Read the model definition and answer for the solid it produces. Units are mm, in the model's axes. Coordinates: 2 decimals unless noted, no trailing zeros. Write each loop counter-clockwise with the first axis right and the second up, starting at its lowest first coordinate (ties: lowest second). Pieces come first, ordered by that corner, then holes. Notation, with made-up numbers: (-2, -29) -> (14, -29) arc R18 cw to (14, -16) -> close; hole circle Ø2 at (87.5, 14.5). An arc over 180 degrees is marked (long way). Return JSON: item names as keys, results as strings.
from build123d import *

# Parameters (mm, degrees)
F0_R     = 22.5
F0_R_2   = 4
F1_DEPTH = 6


with BuildPart() as f1:
    # F0 (on Front) → F1 (new body)
    with BuildSketch(Plane.XZ):
        Circle(F0_R)
        with BuildLine():
            ThreePointArc((12.788895, 9.614789), (14.782073, 6.122935), (15.841797, 2.244431))
            ThreePointArc((15.841797, 2.244431), (17.534038, 1.645973), (18.25, 0))
            ThreePointArc((18.25, 0), (17.534038, -1.645973), (15.841797, -2.244431))
            ThreePointArc((15.841797, -2.244431), (14.782073, -6.122935), (12.788895, -9.614789))
            ThreePointArc((12.788895, -9.614789), (13.360861, -10.380078), (13.563708, -11.313708))
            ThreePointArc((13.563708, -11.313708), (12.101088, -13.42144), (9.614789, -12.788895))
            ThreePointArc((9.614789, -12.788895), (6.122935, -14.782073), (2.244431, -15.841797))
            ThreePointArc((2.244431, -15.841797), (2.248607, -15.920849), (2.25, -16))
            ThreePointArc((2.25, -16), (-0.079151, -18.248607), (-2.244431, -15.841797))
            ThreePointArc((-2.244431, -15.841797), (-6.122935, -14.782073), (-9.614789, -12.788895))
            ThreePointArc((-9.614789, -12.788895), (-12.904699, -12.904699), (-12.788895, -9.614789))
            ThreePointArc((-12.788895, -9.614789), (-14.782073, -6.122935), (-15.841797, -2.244431))
            ThreePointArc((-15.841797, -2.244431), (-18.25, 0), (-15.841797, 2.244431))
            ThreePointArc((-15.841797, 2.244431), (-14.782073, 6.122935), (-12.788895, 9.614789))
            ThreePointArc((-12.788895, 9.614789), (-12.904699, 12.904699), (-9.614789, 12.788895))
            ThreePointArc((-9.614789, 12.788895), (-6.122935, 14.782073), (-2.244431, 15.841797))
            ThreePointArc((-2.244431, 15.841797), (-0.079151, 18.248607), (2.25, 16))
            ThreePointArc((2.25, 16), (2.248607, 15.920849), (2.244431, 15.841797))
            ThreePointArc((2.244431, 15.841797), (6.122935, 14.782073), (9.614789, 12.788895))
            ThreePointArc((9.614789, 12.788895), (12.101088, 13.42144), (13.563708, 11.313708))
            ThreePointArc((13.563708, 11.313708), (13.360861, 10.380078), (12.788895, 9.614789))
        make_face(mode=Mode.SUBTRACT)
        with BuildLine():
            ThreePointArc((15.841797, -2.244431), (13.75, 0), (15.841797, 2.244431))
            ThreePointArc((15.841797, 2.244431), (14.782073, 6.122935), (12.788895, 9.614789))
            ThreePointArc((12.788895, 9.614789), (9.722718, 9.722718), (9.614789, 12.788895))
            ThreePointArc((9.614789, 12.788895), (6.122935, 14.782073), (2.244431, 15.841797))
            ThreePointArc((2.244431, 15.841797), (0, 13.75), (-2.244431, 15.841797))
            ThreePointArc((-2.244431, 15.841797), (-6.122935, 14.782073), (-9.614789, 12.788895))
            ThreePointArc((-9.614789, 12.788895), (-9.205977, 12.101088), (-9.063708, 11.313708))
            ThreePointArc((-9.063708, 11.313708), (-10.380078, 9.266556), (-12.788895, 9.614789))
            ThreePointArc((-12.788895, 9.614789), (-14.782073, 6.122935), (-15.841797, 2.244431))
            ThreePointArc((-15.841797, 2.244431), (-14.354027, 1.534038), (-13.75, 0))
            ThreePointArc((-13.75, 0), (-14.354027, -1.534038), (-15.841797, -2.244431))
            ThreePointArc((-15.841797, -2.244431), (-14.782073, -6.122935), (-12.788895, -9.614789))
            ThreePointArc((-12.788895, -9.614789), (-10.380078, -9.266556), (-9.063708, -11.313708))
            ThreePointArc((-9.063708, -11.313708), (-9.205977, -12.101088), (-9.614789, -12.788895))
            ThreePointArc((-9.614789, -12.788895), (-6.122935, -14.782073), (-2.244431, -15.841797))
            ThreePointArc((-2.244431, -15.841797), (0, -13.75), (2.244431, -15.841797))
            ThreePointArc((2.244431, -15.841797), (6.122935, -14.782073), (9.614789, -12.788895))
            ThreePointArc((9.614789, -12.788895), (9.722718, -9.722718), (12.788895, -9.614789))
            ThreePointArc((12.788895, -9.614789), (14.782073, -6.122935), (15.841797, -2.244431))
        make_face()
        Circle(F0_R_2, mode=Mode.SUBTRACT)
    extrude(amount=F1_DEPTH)


solid = f1.part
1. For a pull along Z with two mould halves and no side action, classify faces 1 (the face through (-9.2, -2.96, -12.09)), 2 (the face through (0, -6, -5)), 3 (the face through (10.382, -2.958, -19.961)), 4 (the face through (-9.21, -2.96, 12.11)) as +Z half, -Z half, draft (parallel to the pull), parting line (faces both ways), or undercut.
Taken from the geometry:
{"face 1": "undercut", "face 2": "draft", "face 3": "parting line", "face 4": "undercut"}
2. Consider L1, parallel to Z at x = 0, y = -1.85; L2, parallel to X at y = -0.9, z = 12; L3, parallel to X at y = -2.3, z = -1. Determine where each line is inside the solid, lowest interval first.
Taken from the geometry:
{"L1": "z = -22.5 to -18.25, -13.75 to -4, 4 to 13.75, 18.25 to 22.5", "L2": "x = -19.03 to -13.46, -9.17 to 9.17, 13.46 to 19.03", "L3": "x = -22.48 to -18.02, -13.98 to -3.87, 3.87 to 13.98, 18.02 to 22.48"}
3. The part is cut by section A-A (x = 0). Determine the outline of the cut face in (y, z), then the cut area to 3 significant figures.
Taken from the geometry:
{"outline": "(-6, -22.5) -> (0, -22.5) -> (0, -18.25) -> (-6, -18.25) -> close; (-6, -13.75) -> (0, -13.75) -> (0, -4) -> (-6, -4) -> close; (-6, 4) -> (0, 4) -> (0, 13.75) -> (-6, 13.75) -> close; (-6, 18.25) -> (0, 18.25) -> (0, 22.5) -> (-6, 22.5) -> close", "area": "168 mm2"}
4. The part is cut by section D-D (z = 15). Determine the outline of the cut face in (x, y).
Taken from the geometry:
{"outline": "(-16.77, -6) -> (-2.02, -6) -> (-2.02, 0) -> (-16.77, 0) -> close; (2.02, -6) -> (16.77, -6) -> (16.77, 0) -> (2.02, 0) -> close"}
5. Flat-ended cylindrical pins translate along their axes: pin 1 Ø7 at (x, z) = (0, 0) entering from +Y; pin 2 Ø1 at (y, z) = (-2, -16) entering from +X; pin 3 Ø2 at (x, y) = (0.5, -2.5) entering from +Z. Find the tip coordinate at first contact, or state that the pin passes through.
Taken from the geometry:
{"pin 1": "passes through", "pin 2": "stops at x = 16.31", "pin 3": "stops at z = 22.5"}
6. The part is cut by section C-C (x = 14.5). Determine the outline of the cut face in (y, z), then the cut area to 3 significant figures.
Taken from the geometry:
{"outline": "(-6, -17.2) -> (0, -17.2) -> (0, -1.68) -> (-6, -1.68) -> close; (-6, 1.68) -> (0, 1.68) -> (0, 17.2) -> (-6, 17.2) -> close", "area": "186 mm2"}
7. The part is cut by section B-B (y = -4.7). Count the separate pieces of the cut face and the enclosed holes in it, then the cut area to 3 significant figures.
Taken from the geometry:
{"separate pieces": "1", "enclosed holes": "9", "area": "1,410 mm2"}
